```python
from build123d import *

# Parameters (mm, degrees)
SKETCH_1_R           = 0.98
EXTRUDE_1_DEPTH      = 5.8
SKETCH_2_W           = 0.5
SKETCH_2_H           = 0.8
EXTRUDE_2_DEPTH      = 3.32
CHAMFER_2_SIZE       = 0.2
EXTRUDE_3_DEPTH      = 1.38
EXTRUDE_3_DEPTH_BACK = 1.38
EXTRUDE_4_DEPTH      = 0.2
EXTRUDE_4_DEPTH_BACK = 0.2
SKETCH_4_R           = 0.25


with BuildPart() as part:
    # 草图1 → 凸台-拉伸1 (new body)
    with BuildSketch(Plane.XY):
        Polygon((0, 0), (6.14, 0), (6.14, 1.9), (6.36, 2.12), (6.36, 4.12), (6.14, 4.34), (6.14, 8.52), (6.36, 8.74), (6.36, 10.74), (6.14, 10.96), (6.14, 12.86), (0, 12.86), align=None)
        with Locations((4.88, 9.74)):
            Circle(SKETCH_1_R, mode=Mode.SUBTRACT)
        with Locations(Location((4.88, 3.12, 0), (0, 0, 180))):
            Circle(SKETCH_1_R, mode=Mode.SUBTRACT)
    extrude(amount=EXTRUDE_1_DEPTH)

    # 草图2 → 凸台-拉伸2 (add)
    with BuildSketch(Plane(origin=(6.14, 0, 0), x_dir=(0, 0, -1), z_dir=(1, 0, 0))):
        with Locations((-2.9, 11.53)):
            Rectangle(SKETCH_2_W, SKETCH_2_H)
        with Locations((-2.9, 1.33)):
            Rectangle(SKETCH_2_W, SKETCH_2_H)
        with Locations((-2.9, 6.43)):
            Rectangle(SKETCH_2_W, SKETCH_2_H)
    extrude(amount=EXTRUDE_2_DEPTH)

    # 倒角2
    chamfer_2_edges = [part.edges().sort_by_distance(p)[0] for p in [
        (9.46, 11.13, 2.9),
        (9.46, 11.93, 2.9),
        (9.46, 0.93, 2.9),
        (9.46, 1.73, 2.9),
        (9.46, 6.03, 2.9),
        (9.46, 6.83, 2.9),
    ]]
    chamfer(chamfer_2_edges, length=CHAMFER_2_SIZE)

    # 草图3 → 凸台-拉伸3 (add, two sides: drawn at the far end of the back side and taken through both)
    with BuildSketch(Plane.XY.offset(2.9).offset(-EXTRUDE_3_DEPTH_BACK)):
        with BuildLine():
            Line((0, 4.8), (-0.5, 4.8))
            ThreePointArc((-0.5, 4.8), (-1, 4.3), (-0.5, 3.8))
            Line((-0.5, 3.8), (0, 3.8))
            Line((0, 3.8), (0, 4.8))
        make_face()
    extrude(amount=EXTRUDE_3_DEPTH + EXTRUDE_3_DEPTH_BACK)

    # 草图4 → 凸台-拉伸4 (add, two sides: drawn at the far end of the back side and taken through both)
    with BuildSketch(Plane.XY.offset(2.9).offset(-EXTRUDE_4_DEPTH_BACK)):
        with Locations((0, 1.93)):
            Circle(SKETCH_4_R)
    extrude(amount=EXTRUDE_4_DEPTH + EXTRUDE_4_DEPTH_BACK)


solid = part.part
```
Work out the finished part from the listing and answer in its coordinate system (mm). A direction names the side the tool comes from. Give positions to 0.01 mm unless a question says otherwise; leave off trailing zeros. Write each loop counter-clockwise with the first axis right and the second up, starting at its lowest first coordinate (ties: lowest second). Pieces come first, ordered by that corner, then holes. Notation, with made-up numbers: (-21.75, 25.5) -> (-16.75, 25.5) arc R34 cw to (-16.75, 55.5) -> close; hole circle Ø1 at (84.25, -27.75). An arc over 180 degrees is marked (long way). Write item = value, one per line.
Q1. Section A-A on y = 9.74 is taken. Determine the outline of the cut face in (x, z).
Computed values:
outline = (0, 0) -> (3.9, 0) -> (3.9, 5.8) -> (0, 5.8) -> close; (5.86, 0) -> (6.36, 0) -> (6.36, 5.8) -> (5.86, 5.8) -> close
Q2. Section B-B on z = 1.75 is taken. Determine the outline of the cut face in (x, y).
Computed values:
outline = (-0.5, 3.8) -> (0, 3.8) -> (0, 0) -> (6.14, 0) -> (6.14, 1.9) -> (6.36, 2.12) -> (6.36, 4.12) -> (6.14, 4.34) -> (6.14, 8.52) -> (6.36, 8.74) -> (6.36, 10.74) -> (6.14, 10.96) -> (6.14, 12.86) -> (0, 12.86) -> (0, 4.8) -> (-0.5, 4.8) arc R0.5 ccw to start; hole circle Ø1.96 at (4.88, 3.12); hole circle Ø1.96 at (4.88, 9.74)
Q3. A tool of negligible diameter and unlimited length cuts with its end or side. For faces 5 (the flat face through (-0.5, 4.3, 4.28)), 6 (the cylindrical face through (5.602, 2.458, 2.859)), 7 (the flat face through (-0.5, 4.3, 1.52)), from which of +Z, -Z, +X, -X, +Y, -Y can it reach the whole face along a straight path? Write none if from no direction.
Computed values:
face_5 = +Z, -X, +Y, -Y
face_6 = +Z, -Z
face_7 = -Z, -X, +Y, -Y
Q4. Consider line 1 along Y through (x, z) = (4.88, 3.75); line 2 along X through (y, z) = (3.12, 4.35); line 3 along Y through (x, z) = (5.75, 5). Determine where each line is inside the solid, lowest interval first.
Computed values:
line_1 = 0 to 2.14, 4.1 to 8.76, 10.72 to 12.86
line_2 = 0 to 3.9, 5.86 to 6.36
line_3 = 0 to 2.67, 3.57 to 9.29, 10.19 to 12.86
Q5. Flat-ended cylindrical pins translate along their axes: pin 1 Ø1 at (x, y) = (7, 2.5) entering from -Z; pin 2 Ø0.6 at (x, y) = (7.5, 11.5) entering from +Z; pin 3 Ø1.5 at (y, z) = (7.5, 3.5) entering from -X; pin 4 Ø1.5 at (y, z) = (4, 3.5) entering from +X. Find the tip coordinate at first contact, or state that the pin passes through.
Computed values:
pin_1 = through
pin_2 = 3.15
pin_3 = 0
pin_4 = 6.36
Q6. Section C-C on x = 4.88 is taken. Determine the outline of the cut face in (y, z).
Computed values:
outline = (0, 0) -> (2.14, 0) -> (2.14, 5.8) -> (0, 5.8) -> close; (4.1, 0) -> (8.76, 0) -> (8.76, 5.8) -> (4.1, 5.8) -> close; (10.72, 0) -> (12.86, 0) -> (12.86, 5.8) -> (10.72, 5.8) -> close
Q7. Section D-D on z = 0.55 is taken. Determine the outline of the cut face in (x, y), and give its area (3 significant figures).
Computed values:
outline = (0, 0) -> (6.14, 0) -> (6.14, 1.9) -> (6.36, 2.12) -> (6.36, 4.12) -> (6.14, 4.34) -> (6.14, 8.52) -> (6.36, 8.74) -> (6.36, 10.74) -> (6.14, 10.96) -> (6.14, 12.86) -> (0, 12.86) -> close; hole circle Ø1.96 at (4.88, 3.12); hole circle Ø1.96 at (4.88, 9.74)
area = 73.9 mm^2
Q8. For a pull along Y with two mould halves and no side action, classify faces 1 (the flat face through (3, 0, 3)), 2 (the cylindrical face through (4.75, 10.71, 2.86)), 3 (the flat face through (3, 7, 0)), 4 (the cylindrical face through (-1, 4.3, 2.9)) as pulls with the +Y half, pulls with the -Y half, needs draft (parallel to the pull), parting line crosses it, or undercut.
Computed values:
face_1 = pulls with the -Y half
face_2 = undercut
face_3 = needs draft
face_4 = parting line crosses it
